from build123d import *

# Parameters (mm, degrees)
BOSS_EXTRUDE1_DEPTH = 6
CHAMFER1_SIZE       = 0.5


with BuildPart() as part:
    # Sketch1 → Boss-Extrude1 (new body)
    with BuildSketch(Plane(origin=(0, 0, 0), x_dir=(1, 0, 0), z_dir=(0, 1, 0))):
        Polygon((8, 0), (6.92820323, 4), (4, 6.92820323), (0, 8), (-4, 6.92820323), (-6.92820323, 4), (-8, 0), (-6.92820323, -4), (-4, -6.92820323), (0, -8), (4, -6.92820323), (6.92820323, -4), align=None)
        Polygon((2.976578551, 0), (2.104758878, 2.104758878), (0, 2.976578551), (-2.104758878, 2.104758878), (-2.976578551, 0), (-2.104758878, -2.104758878), (0, -2.976578551), (2.104758878, -2.104758878), align=None, mode=Mode.SUBTRACT)
    extrude(amount=BOSS_EXTRUDE1_DEPTH)

    # Chamfer1
    chamfer1_edges = [part.edges().sort_by_distance(p)[0] for p in [
        (5.464101615, 6, -5.464101615),
        (5.464101615, 0, 5.464101615),
        (2, 0, 7.464101615),
        (-2, 0, 7.464101615),
        (-5.464101615, 0, 5.464101615),
        (-7.464101615, 0, 2),
        (-7.464101615, 0, -2),
        (2, 6, -7.464101615),
        (-5.464101615, 0, -5.464101615),
        (-2, 0, -7.464101615),
        (2, 0, -7.464101615),
        (5.464101615, 0, -5.464101615),
        (7.464101615, 0, -2),
        (7.464101615, 0, 2),
        (-2, 6, -7.464101615),
        (-5.464101615, 6, -5.464101615),
        (-7.464101615, 6, -2),
        (-7.464101615, 6, 2),
        (-5.464101615, 6, 5.464101615),
        (-2, 6, 7.464101615),
        (2, 6, 7.464101615),
        (2.540668714, 0, 1.052379439),
        (2.540668714, 0, -1.052379439),
        (1.052379439, 0, -2.540668714),
        (-1.052379439, 0, -2.540668714),
        (5.464101615, 6, 5.464101615),
        (-2.540668714, 0, -1.052379439),
        (-2.540668714, 0, 1.052379439),
        (-1.052379439, 0, 2.540668714),
        (1.052379439, 0, 2.540668714),
        (2.540668714, 6, 1.052379439),
        (2.540668714, 6, -1.052379439),
        (1.052379439, 6, -2.540668714),
        (-1.052379439, 6, -2.540668714),
        (7.464101615, 6, 2),
        (-2.540668714, 6, -1.052379439),
        (-2.540668714, 6, 1.052379439),
        (-1.052379439, 6, 2.540668714),
        (1.052379439, 6, 2.540668714),
        (7.464101615, 6, -2),
    ]]
    chamfer(chamfer1_edges, length=CHAMFER1_SIZE)


solid = part.part
Geometry check sheet. Reference: the model listing, model coordinates, mm. A direction names the side the tool comes from. Round coordinates to 2 decimals unless told otherwise and drop trailing zeros. Loops run counter-clockwise (first coordinate to the right, second up) from the corner with the lowest first, then second, coordinate; pieces in that order, holes last. Notation, with made-up numbers: (42, 79.25) -> (50, 79.25) arc R20 cw to (50, 83.25) -> close; hole circle Ø1 at (77, -20.75). An arc over 180 degrees is marked (long way). Answer as a JSON object with one key per item and string values. Group by question number.
Item 1: Set-up check for faces 4 (the face through (-2.78, 5.75, 1.13)), 5 (the face through (-5.485, 2.965, 5.444)): record each of +Z, -Z, +X, -X, +Y, -Y from which the full face is reachable in a straight line by a thin tool's end or side.
Item 2: Cross-section at B-B, the plane y = 2.25. Record the cut outline in (x, z), plus the area to 3 significant figures.
Item 3: Cross-section at C-C, the plane x = 1.5. Record the cut outline in (y, z).
Item 4: Release check for a two-part mould opening along Z. For faces 1 (the face through (-1.167, 0.246, 2.768)), 2 (the face through (7.472, 2.965, -1.972)), 3 (the face through (-2.028, 2.965, 7.457)) record: pulls with the +Z half, pulls with the -Z half, needs draft (parallel to the pull), parting line crosses it, or undercut.
Item 5: Cross-section at D-D, the plane z = 6.25. Record the cut outline in (x, y).
Item 6: Thickness scan on line 1 along X through (y, z) = (1.5, -1.75); line 2 along Z through (x, y) = (-0.25, 2). Record the ranges inside material, lowest first.
Item 7: Cross-section at A-A, the plane z = -1.5. Record the cut outline in (x, y).
Item 8: Depth check by flat-ended pin: pin 1 Ø3 at (x, y) = (-4, 0.5) entering from -Z; pin 2 Ø2 at (y, z) = (2, 4.5) entering from -X. Enter the tip coordinate at first touch or a pass-through.
Determined:
{
 "1": {"face 4": "+Y", "face 5": "+Z, -X, +Y, -Y"},
 "2": {"outline": "(-8, 0) -> (-6.93, -4) -> (-4, -6.93) -> (0, -8) -> (4, -6.93) -> (6.93, -4) -> (8, 0) -> (6.93, 4) -> (4, 6.93) -> (0, 8) -> (-4, 6.93) -> (-6.93, 4) -> close; hole (-2.98, 0) -> (-2.1, -2.1) -> (0, -2.98) -> (2.1, -2.1) -> (2.98, 0) -> (2.1, 2.1) -> (0, 2.98) -> (-2.1, 2.1) -> close", "area": "167 mm²"},
 "3": {"outline": "(0, -7.08) -> (0.5, -7.6) -> (5.5, -7.6) -> (6, -7.08) -> (6, -2.9) -> (5.5, -2.36) -> (0.5, -2.36) -> (0, -2.9) -> close; (0, 2.9) -> (0.5, 2.36) -> (5.5, 2.36) -> (6, 2.9) -> (6, 7.08) -> (5.5, 7.6) -> (0.5, 7.6) -> (0, 7.08) -> close"},
 "4": {"face 1": "undercut", "face 2": "pulls with the -Z half", "face 3": "pulls with the +Z half"},
 "5": {"outline": "(-4.68, 0.5) -> (-3.97, 0) -> (3.97, 0) -> (4.68, 0.5) -> (4.68, 5.5) -> (3.97, 6) -> (-3.97, 6) -> (-4.68, 5.5) -> close"},
 "6": {"line 1": "x = -7.53 to -2.25, 2.25 to 7.53", "line 2": "z = -7.93 to -2.87, 2.87 to 7.93"},
 "7": {"outline": "(-7.6, 0.5) -> (-7.08, 0) -> (-2.9, 0) -> (-2.36, 0.5) -> (-2.36, 5.5) -> (-2.9, 6) -> (-7.08, 6) -> (-7.6, 5.5) -> close; (2.36, 0.5) -> (2.9, 0) -> (7.08, 0) -> (7.6, 0.5) -> (7.6, 5.5) -> (7.08, 6) -> (2.9, 6) -> (2.36, 5.5) -> close"},
 "8": {"pin 1": "stops at z = -7.33", "pin 2": "stops at x = -7.06"}
}
